from build123d import *

# Parameters (mm, degrees)
SKETCH_1_W      = 40
SKETCH_1_H      = 40
EXTRUDE_1_DEPTH = 40
SKETCH_2_R      = 20
EXTRUDE_2_DEPTH = 35
SKETCH_8_R      = 3.439176188
EXTRUDE_3_DEPTH = 5
FILLET_3_R      = 0.5
CHAMFER_1_SIZE  = 0.5
CHAMFER_2_SIZE  = 2
CHAMFER_3_SIZE  = 2
SKETCH_9_R      = 0.5
EXTRUDE_4_DEPTH = 300


with BuildPart() as part:
    # 草图1 → 凸台-拉伸1 (new body)
    with BuildSketch(Plane.XY):
        Rectangle(SKETCH_1_W, SKETCH_1_H)
    extrude(amount=EXTRUDE_1_DEPTH)

    # 草图2 → 凸台-拉伸2 (add)
    with BuildSketch(Plane.XY.offset(40)):
        Circle(SKETCH_2_R)
    extrude(amount=EXTRUDE_2_DEPTH)

    # 草图8 → 凸台-拉伸3 (add)
    with BuildSketch(Plane(origin=(0, 0, 0), x_dir=(-1, 0, 0), z_dir=(0, 0, -1))):
        with Locations((8.63222484, 8.081848089)):
            Circle(SKETCH_8_R)
    extrude(amount=EXTRUDE_3_DEPTH)

    # 圆角3
    fillet_3_edges = [part.edges().sort_by_distance(p)[0] for p in [
        (-5.193048652, 8.081848089, 0),
    ]]
    fillet(fillet_3_edges, radius=FILLET_3_R)

    # 倒角1
    chamfer_1_edges = [part.edges().sort_by_distance(p)[0] for p in [
        (-5.193048652, 8.081848089, -5),
    ]]
    chamfer(chamfer_1_edges, length=CHAMFER_1_SIZE)

    # 倒角2
    chamfer_2_edges = [part.edges().sort_by_distance(p)[0] for p in [
        (-20, 20, 20),
        (20, 20, 20),
        (20, -20, 20),
        (-20, -20, 20),
    ]]
    chamfer(chamfer_2_edges, length=CHAMFER_2_SIZE)

    # 倒角3
    chamfer_3_edges = [part.edges().sort_by_distance(p)[0] for p in [
        (-20, 0, 75),
    ]]
    chamfer(chamfer_3_edges, length=CHAMFER_3_SIZE)

    # 草图9 → 凸台-拉伸4 (add)
    with BuildSketch(Plane.XY.offset(75)):
        Circle(SKETCH_9_R)
    extrude(amount=EXTRUDE_4_DEPTH)


solid = part.part
Here's how the part is built. I have some questions about the finished solid (model axes, mm). A direction names the side the tool comes from. Round coordinates to 2 decimals unless told otherwise and drop trailing zeros. Order: outer loops, then holes, each group sorted by start corner. A loop starts at its lowest first (then second) coordinate and runs counter-clockwise, first axis right, second up. Notation, with made-up numbers: (-5.5, 30) -> (22.5, 30) arc R23 cw to (22.5, 62) -> close; hole circle Ø3 at (-35, 53). An arc over 180 degrees is marked (long way). Return JSON: item names as keys, results as strings.
Q1. Which directions (+Z, -Z, +X, -X, +Y, -Y) give clear straight access to the entire face, cutting with the end or side of a thin tool? Please do faces 1 (the cylindrical face through (-4.336, -19.524, 56.269)), 2 (the flat face through (-16, -15, 40)), 3 (the cylindrical face through (-11.913, 9.115, -2.472)), 4 (the flat face through (15, 15, 40)).
Filled sheet:
{"face 1": "+Z", "face 2": "+Z, -X, -Y", "face 3": "-Z", "face 4": "+Z, +X, +Y"}
Q2. If we section it at A-A on z = 159: List the corners of the cut face in (x, y) for me.
Filled sheet:
{"outline": "circle Ø1 at (0, 0)"}
Q3. For pin 1 Ø5 at (x, y) = (-2.5, 3.5) entering from +Z; pin 2 Ø3 at (x, z) = (1.5, 300.5) entering from -Y; pin 3 Ø1.5 at (x, y) = (14, -9) entering from -Z, each with a flat end and sliding along its axis, tell me the tip position at first contact or that it passes through.
Filled sheet:
{"pin 1": "stops at z = 75", "pin 2": "stops at y = -0.5", "pin 3": "stops at z = 0"}
Q4. I need wall thicknesses on line 1 along Z through (x, y) = (6, 12); line 2 along Z through (x, y) = (-11, 9). Which ranges of each line are inside material? Lowest first, please. Write a range as from..to.
Filled sheet:
{"line 1": "z = 0..75", "line 2": "z = -5..75"}
